Check sheet for the modelled part. Datum: model origin and axes. Units: mm. A direction names the side the tool comes from. Give positions to 0.01 mm unless a question says otherwise; leave off trailing zeros. Loops run counter-clockwise (first coordinate to the right, second up) from the corner with the lowest first, then second, coordinate; pieces in that order, holes last. Notation, with made-up numbers: (-30, 81) - (20, 81) arc R22 cw to (20, 91) - close; hole circle Ø5 at (-20.5, -19.75). An arc over 180 degrees is marked (long way). Use one line per item in the form item = value.
from build123d import *

# Parameters (mm, degrees)
BOX_W        = 1
BOX_H        = 6
BOX_DEPTH    = 6
SKETCH001_R  = 3.5
POCKET_DEPTH = 3
FILLET_R     = 0.2
FILLET001_R  = 0.2


with BuildPart() as cube:
    # Box → Box (new body)
    with BuildSketch(Plane(origin=(-0.5, 0, -3), x_dir=(1, 0, 0), z_dir=(0, 0, 1))):
        with Locations((0.5, 3)):
            Rectangle(BOX_W, BOX_H)
    extrude(amount=BOX_DEPTH)


with BuildPart() as cut:
    # Sketch → Revolution (revolve)
    with BuildSketch(Plane.XZ):
        with BuildLine():
            Line((5.4, 3.5), (5.4, 3))
            Line((5.4, 3), (4.4, 3))
            Line((4.4, 3), (4.4, 0))
            Line((4.4, 0), (0, 0))
            Line((0, 0), (0, 4))
            Line((0, 4), (3.5, 4))
            ThreePointArc((5.4, 3.5), (4.482344, 3.872908), (3.5, 4))
        make_face()
    revolve(axis=Axis((0, 0, 0), (0, 0, 1)))

    # Sketch001 (on Face4 of Revolution) → Pocket (cut)
    with BuildSketch(Plane(origin=(0, 0, 0), x_dir=(1, 0, 0), z_dir=(0, 0, -1))):
        Circle(SKETCH001_R)
    extrude(amount=-POCKET_DEPTH, mode=Mode.SUBTRACT)

    # Fillet
    fillet_edges = [cut.edges().sort_by_distance(p)[0] for p in [
        (-4.4, 0, 0),
    ]]
    fillet(fillet_edges, radius=FILLET_R)

    # Fillet001
    fillet001_edges = [cut.edges().sort_by_distance(p)[0] for p in [
        (-3.5, 0, 0),
    ]]
    fillet(fillet001_edges, radius=FILLET001_R)

    # Cut: cut Cube
    add(cube.part, mode=Mode.SUBTRACT)


solid = cut.part
Item 1: Section check A-A on z = 0.75. Record the boundary of the cut face in (x, y), then the cut area to 3 significant figures.
Answer block:
outline = (-0.5, 3.46) - (-0.5, 4.37) arc R4.4 ccw (long way) to (0.5, 4.37) - (0.5, 3.46) arc R3.5 cw (long way) to start
area = 21.4 mm2
Item 2: Mould release check, pull along Y, two halves, no side actions. Record for faces 4 (the face through (-0.186, -4.396, 1.58)), 5 (the face through (0.5, 4, 1)), 6 (the face through (0.1, -3.5, 1.6)): released by +Y, released by -Y, zero draft, split by the parting line, or undercut.
Answer block:
face_4 = split by the parting line
face_5 = zero draft
face_6 = undercut
Item 3: Access from +Z, -Z, +X, -X, +Y, -Y to the whole of each face (thin tool, end or side, straight path). Record for faces 1 (the face through (0, 0, 3)), 2 (the face through (-0.5, 4, 1)), 3 (the face through (0, 0, 4)).
Answer block:
face_1 = -Z
face_2 = -Z, +Y
face_3 = +Z, +X, -X, +Y, -Y
Item 4: Gauge pin test, flat ends, axial feed: P1, Ø6, axis at x = -4, y = 0.5, coming from the -Z side; P2, Ø1, axis at y = 4, z = 1.5, coming from the +X side; P3, Ø0.5, axis at y = 4, z = 2, coming from the -X side. Record the tip position at first contact, or that the pin passes through.
Answer block:
P1 = 0
P2 = 2.67
P3 = -2.3
Item 5: Thickness scan on L1, parallel to X at y = 0, z = 2; L2, parallel to Y at x = 0, z = 2.35; L3, parallel to Z at x = 0.75, y = -2.75. Record the ranges inside material, lowest first.
Answer block:
L1 = -4.4 to -3.5, 3.5 to 4.4
L2 = -4.4 to -3.5
L3 = 3 to 4
